```python
from build123d import *

# Parameters (mm, degrees)
F1_DEPTH  = 8
F3_DEPTH  = 8
F5_DEPTH  = 25
F7_DEPTH  = 25
F9_DEPTH  = 25
F11_DEPTH = 8
F13_DEPTH = 25
F14_R     = 6.3379866709
F14_R_2   = 4
F14_R_3   = 6.8285415101
F14_R_4   = 3.5
F14_R_5   = 5.2949091489
F14_R_6   = 3
F15_DEPTH = 8
F16_R     = 4
F16_R_2   = 3.5
F16_R_3   = 3
F17_DEPTH = 25
F18_R     = 6.5
F18_R_2   = 6
F19_DEPTH = 25
F20_R     = 6.5
F20_R_2   = 5
F21_DEPTH = 25
F22_R     = 6
F22_R_2   = 5
F23_DEPTH = 8
F24_R     = 9.6843488415
F24_R_2   = 6.5
F25_DEPTH = 8
F26_R     = 6.5
F26_R_2   = 6
F27_DEPTH = 8
F29_DEPTH = 25
F30_SIZE  = 2


with BuildPart() as f1:
    # F0 (on Front) → F1 (new body)
    with BuildSketch(Plane.XZ):
        Polygon((-70, -74.8061388731), (0, -74.8061388731), (0, 65.1938611269), align=None)
    extrude(amount=F1_DEPTH)

    # F2 (on face) → F3 (join)
    with BuildSketch(Plane.XZ.offset(8)):
        Polygon((-70, -74.8061388731), (0, 65.1938611269), (0, 115.1938611269), align=None)
    extrude(amount=-F3_DEPTH)

    # F4 (on face) → F5 (cut)
    with BuildSketch(Plane.XZ.offset(8)):
        Polygon((0, 65.1938611269), (0, 115.1938611269), (-70, -74.8061388731), align=None)
    extrude(amount=-F5_DEPTH, mode=Mode.SUBTRACT)

    # F6 (on face) → F7 (cut)
    with BuildSketch(Plane.XZ.offset(8)):
        with BuildLine():
            Line((-10, -59.8061388731), (-10, -64.8061388731))
            ThreePointArc((-10, -64.8061388731), (-6.4644660941, -63.341672779), (-5, -59.8061388731))
            ThreePointArc((-5, -59.8061388731), (-6.4644660941, -56.2706049672), (-10, -54.8061388731))
            Line((-10, -54.8061388731), (-10, -59.8061388731))
        make_face()
        with BuildLine():
            ThreePointArc((-10, -54.8061388731), (-15, -59.8061388731), (-10, -64.8061388731))
            Line((-10, -64.8061388731), (-10, -59.8061388731))
            Line((-10, -59.8061388731), (-10, -54.8061388731))
        make_face()
        with BuildLine():
            Line((-10, -38.8061388731), (-10, -42.8061388731))
            ThreePointArc((-10, -42.8061388731), (-7.1715728753, -41.6345659978), (-6, -38.8061388731))
            ThreePointArc((-6, -38.8061388731), (-7.1715728753, -35.9777117484), (-10, -34.8061388731))
            Line((-10, -34.8061388731), (-10, -38.8061388731))
        make_face()
        with BuildLine():
            ThreePointArc((-10, -34.8061388731), (-14, -38.8061388731), (-10, -42.8061388731))
            Line((-10, -42.8061388731), (-10, -38.8061388731))
            Line((-10, -38.8061388731), (-10, -34.8061388731))
        make_face()
        with BuildLine():
            Line((-10, -19.3061388731), (-10, -22.8061388731))
            ThreePointArc((-10, -22.8061388731), (-7.5251262658, -21.7810126073), (-6.5, -19.3061388731))
            ThreePointArc((-6.5, -19.3061388731), (-7.5251262658, -16.8312651389), (-10, -15.8061388731))
            Line((-10, -15.8061388731), (-10, -19.3061388731))
        make_face()
        with BuildLine():
            ThreePointArc((-10, -15.8061388731), (-13.5, -19.3061388731), (-10, -22.8061388731))
            Line((-10, -22.8061388731), (-10, -19.3061388731))
            Line((-10, -19.3061388731), (-10, -15.8061388731))
        make_face()
        with BuildLine():
            ThreePointArc((-7, -0.8061388731), (-12.1213203436, 1.3151814705), (-10, -3.8061388731))
            ThreePointArc((-10, -3.8061388731), (-7.8786796564, -2.9274592167), (-7, -0.8061388731))
        make_face()
    extrude(amount=-F7_DEPTH, mode=Mode.SUBTRACT)

    # F8 (on face) → F9 (cut)
    with BuildSketch(Plane.XZ.offset(8)):
        Polygon((0, 35.1938611269), (0, 65.1938611269), (-70, -74.8061388731), align=None)
    extrude(amount=-F9_DEPTH, mode=Mode.SUBTRACT)

    # F10 (on face) → F11 (join)
    with BuildSketch(Plane.XZ.offset(8)):
        Polygon((5, 43.051003984), (0, 35.1938611269), (0, -74.8061388731), (5, -74.8061388731), align=None)
    extrude(amount=-F11_DEPTH)

    # F12 (on face) → F13 (cut)
    with BuildSketch(Plane.XZ.offset(8)):
        Polygon((5, 43.051003984), (-70, -74.8061388731), (-65, -74.8061388731), align=None)
    extrude(amount=-F13_DEPTH, mode=Mode.SUBTRACT)

    # F14 (on face) → F15 (join)
    with BuildSketch(Plane.XZ.offset(8)):
        with Locations((-10, -38.8061388731)):
            Circle(F14_R)
        with Locations((-10, -38.8061388731)):
            Circle(F14_R_2, mode=Mode.SUBTRACT)
        with Locations((-10, -38.8061388731)):
            Circle(F14_R_2)
        with Locations((-10, -19.3061388731)):
            Circle(F14_R_3)
        with Locations((-10, -19.3061388731)):
            Circle(F14_R_4, mode=Mode.SUBTRACT)
        with Locations((-10, -19.3061388731)):
            Circle(F14_R_4)
        with Locations((-10, -0.8061388731)):
            Circle(F14_R_5)
        with Locations((-10, -0.8061388731)):
            Circle(F14_R_6, mode=Mode.SUBTRACT)
        with Locations((-10, -0.8061388731)):
            Circle(F14_R_6)
    extrude(amount=-F15_DEPTH)

    # F16 (on face) → F17 (cut)
    with BuildSketch(Plane.XZ.offset(8)):
        with Locations((-9, -38.8061388731)):
            Circle(F16_R)
        with Locations((-8.5, -19.3061388731)):
            Circle(F16_R_2)
        with Locations((-8, -0.8061388731)):
            Circle(F16_R_3)
    extrude(amount=-F17_DEPTH, mode=Mode.SUBTRACT)

    # F18 (on face) → F19 (cut)
    with BuildSketch(Plane.XZ.offset(8)):
        with Locations((-31.5, -59.8061388731)):
            Circle(F18_R)
        with Locations((-29, -38.8061388731)):
            Circle(F18_R_2)
    extrude(amount=-F19_DEPTH, mode=Mode.SUBTRACT)

    # F20 (on face) → F21 (cut)
    with BuildSketch(Plane.XZ.offset(8)):
        with Locations((-10, -59.8061388731)):
            Circle(F20_R)
        with Locations((-10, -59.8061388731)):
            Circle(F20_R_2, mode=Mode.SUBTRACT)
    extrude(amount=-F21_DEPTH, mode=Mode.SUBTRACT)

    # F22 (on face) → F23 (join)
    with BuildSketch(Plane.XZ.offset(8)):
        with Locations((-29, -38.8061388731)):
            Circle(F22_R)
        with Locations((-29, -38.8061388731)):
            Circle(F22_R_2, mode=Mode.SUBTRACT)
    extrude(amount=-F23_DEPTH)

    # F24 (on face) → F25 (join)
    with BuildSketch(Plane.XZ.offset(8)):
        with Locations((-31.5, -59.8061388731)):
            Circle(F24_R)
        with Locations((-31.5, -59.8061388731)):
            Circle(F24_R_2, mode=Mode.SUBTRACT)
        with Locations((-31.5, -59.8061388731)):
            Circle(F24_R_2)
    extrude(amount=-F25_DEPTH)

    # F26 (on face) → F27 (join)
    with BuildSketch(Plane.XZ.offset(8)):
        with Locations((-10, -59.8061388731)):
            Circle(F26_R)
        with Locations((-10, -59.8061388731)):
            Circle(F26_R_2, mode=Mode.SUBTRACT)
    extrude(amount=-F27_DEPTH)

    # F28 (on face) → F29 (cut)
    with BuildSketch(Plane.XZ.offset(8)):
        with BuildLine():
            ThreePointArc((-33.7916220485, -54.4677933458), (-43.259967738, -62.8182430641), (-31, -59.8061388731))
            Line((-31, -59.8061388731), (-37.5, -59.8061388731))
            Line((-37.5, -59.8061388731), (-33.7916220485, -54.4677933458))
        make_face()
        with BuildLine():
            Line((-37.5, -59.8061388731), (-31, -59.8061388731))
            ThreePointArc((-31, -59.8061388731), (-31.740032262, -56.7940346821), (-33.7916220485, -54.4677933458))
            Line((-33.7916220485, -54.4677933458), (-37.5, -59.8061388731))
        make_face()
    extrude(amount=-F29_DEPTH, mode=Mode.SUBTRACT)

    # F30
    f30_edges = [f1.edges().sort_by_distance(p)[0] for p in [
        (5, -8, -15.877567),
        (-30, -8, -15.877567),
        (-30, -8, -74.806139),
    ]]
    chamfer(f30_edges, length=F30_SIZE)


solid = f1.part
```
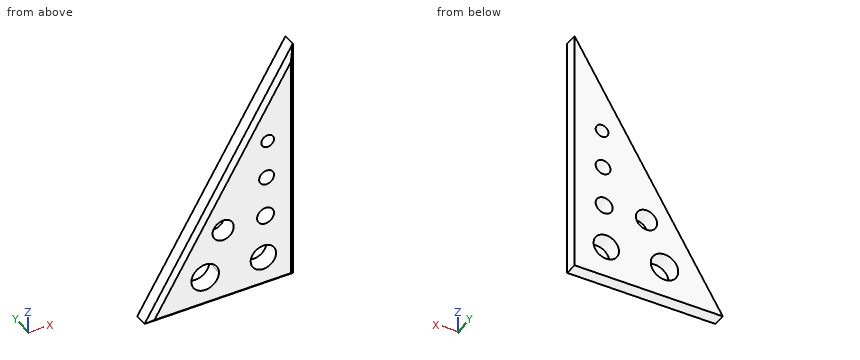
Source: CAD feature listing. Evaluate the final solid. Frame: model axes, mm. Round coordinates to 2 decimals unless told otherwise and drop trailing zeros. Loops run counter-clockwise (first coordinate to the right, second up) from the corner with the lowest first, then second, coordinate; pieces in that order, holes last.
1. Section query D-D on x = -29. Output: boundary loops of the cut face in (y, z), and give its area (3 significant figures).
2. Section query B-B on x = -9. Output: boundary loops of the cut face in (y, z), and give its area (3 significant figures).
3. Section query A-A on x = -37.5. Output: boundary loops of the cut face in (y, z).
4. Section query C-C on z = 17. Output: boundary loops of the cut face in (x, y), and give its area (3 significant figures).
5. Ray query, L1, parallel to X at y = -2.5, z = -59; L2, parallel to Z at x = -9, y = -4.75; L3, parallel to Z at x = -9.5, y = -0.75. Return the intervals inside material, ascending.
6. Contact query for flat-ended pins moving along their axis: pin 1 (3 mm diameter, centred on x = -25, z = -49, fed in from +Y); pin 2 (1 mm diameter, centred on y = -6, z = 14, fed in from -X). Output: stop coordinate, or through.
Answers below:
1. outline: (-8, -72.81) - (-6, -74.81) - (0, -74.81) - (0, -43.81) - (-8, -43.81) - close; (-8, -33.81) - (0, -33.81) - (0, -14.19) - (-6, -14.19) - (-8, -18.11) - close
1. area: 399 mm2
2. outline: (-8, -72.81) - (-6, -74.81) - (0, -74.81) - (0, -65.72) - (-8, -65.72) - close; (-8, -53.89) - (0, -53.89) - (0, -42.81) - (-8, -42.81) - close; (-8, -34.81) - (0, -34.81) - (0, -22.77) - (-8, -22.77) - close; (-8, -15.84) - (0, -15.84) - (0, -3.63) - (-8, -3.63) - close; (-8, 2.02) - (0, 2.02) - (0, 19.48) - (-6, 19.48) - (-8, 15.56) - close
2. area: 489 mm2
3. outline: (-8, -72.81) - (-6, -74.81) - (0, -74.81) - (0, -66.31) - (-8, -66.31) - close; (-8, -53.31) - (0, -53.31) - (0, -28.51) - (-6, -28.51) - (-8, -32.42) - close
4. outline: (-10.47, -6) - (-8.15, -8) - (3, -8) - (5, -6) - (5, 0) - (-10.47, 0) - close
4. area: 119 mm2
5. L1: x = -55.61 to -43.95, -31.05 to -15.95, -4.05 to 5
5. L2: z = -74.81 to -65.72, -53.89 to -42.81, -34.81 to -22.77, -15.84 to -3.63, 2.02 to 19.48
5. L3: z = -74.81 to -65.79, -53.83 to -42.77, -34.84 to -22.66, -15.95 to -3.4, 1.79 to 18.64
6. pin 1: stops at y = 0
6. pin 2: stops at x = -12.55
